For this review, take the finished solid that the model builds, in its own axes (mm). Give positions to 0.01 mm unless a question says otherwise; leave off trailing zeros. Write each loop counter-clockwise with the first axis right and the second up, starting at its lowest first coordinate (ties: lowest second). Pieces come first, ordered by that corner, then holes. Notation, with made-up numbers: M 11.25,38 L 54.25,38 A27 cw 54.25,66 Z; hole C 62,56.5 d9. An arc over 180 degrees is marked long. Write item = value, one per line.
```python
from build123d import *

# Parameters (mm, degrees)
SKETCH_2_W      = 70
SKETCH_2_H      = 70
SKETCH_2_R      = 2.15
EXTRUDE_1_DEPTH = 4
SKETCH_3_R      = 3.5
SKETCH_3_R_2    = 1.5
EXTRUDE_2_DEPTH = 5
FILLET_1_R      = 5


with BuildPart() as part:
    # 草圖2 → 填料-伸長1 (new body)
    with BuildSketch(Plane(origin=(0, 0, 0), x_dir=(1, 0, 0), z_dir=(0, 1, 0))):
        Rectangle(SKETCH_2_W, SKETCH_2_H)
        with Locations(Location((-25, 25, 0), (0, 0, 270))):
            Circle(SKETCH_2_R, mode=Mode.SUBTRACT)
        with Locations(Location((25, 25, 0), (0, 0, 270))):
            Circle(SKETCH_2_R, mode=Mode.SUBTRACT)
        with Locations(Location((-25, -25, 0), (0, 0, 270))):
            Circle(SKETCH_2_R, mode=Mode.SUBTRACT)
        with Locations(Location((25, -25, 0), (0, 0, 270))):
            Circle(SKETCH_2_R, mode=Mode.SUBTRACT)
    extrude(amount=EXTRUDE_1_DEPTH)

    # 草圖3 → 填料-伸長2 (add)
    # profile 1 of 4: a face of its own
    with BuildSketch(Plane(origin=(0, 4, 0), x_dir=(1, 0, 0), z_dir=(0, 1, 0))):
        with Locations(Location((-20, 30, 0), (0, 0, 270))):
            Circle(SKETCH_3_R)
        with Locations(Location((-20, 30, 0), (0, 0, 270))):
            Circle(SKETCH_3_R_2, mode=Mode.SUBTRACT)
    # profile 2 of 4: a face of its own
    with BuildSketch(Plane(origin=(0, 4, 0), x_dir=(1, 0, 0), z_dir=(0, 1, 0))):
        with Locations(Location((30.8, 14.8, 0), (0, 0, 270))):
            Circle(SKETCH_3_R)
        with Locations(Location((30.8, 14.8, 0), (0, 0, 270))):
            Circle(SKETCH_3_R_2, mode=Mode.SUBTRACT)
    # profile 3 of 4: a face of its own
    with BuildSketch(Plane(origin=(0, 4, 0), x_dir=(1, 0, 0), z_dir=(0, 1, 0))):
        with Locations(Location((30.8, -13.1, 0), (0, 0, 270))):
            Circle(SKETCH_3_R)
        with Locations(Location((30.8, -13.1, 0), (0, 0, 270))):
            Circle(SKETCH_3_R_2, mode=Mode.SUBTRACT)
    # profile 4 of 4: a face of its own
    with BuildSketch(Plane(origin=(0, 4, 0), x_dir=(1, 0, 0), z_dir=(0, 1, 0))):
        with Locations(Location((-21.3, -18.2, 0), (0, 0, 270))):
            Circle(SKETCH_3_R)
        with Locations(Location((-21.3, -18.2, 0), (0, 0, 270))):
            Circle(SKETCH_3_R_2, mode=Mode.SUBTRACT)
    extrude(amount=EXTRUDE_2_DEPTH)

    # 圓角1
    fillet_1_edges = [part.edges().sort_by_distance(p)[0] for p in [
        (35, 2, 35),
        (-35, 2, 35),
        (-35, 2, -35),
        (35, 2, -35),
    ]]
    fillet(fillet_1_edges, radius=FILLET_1_R)


solid = part.part
```
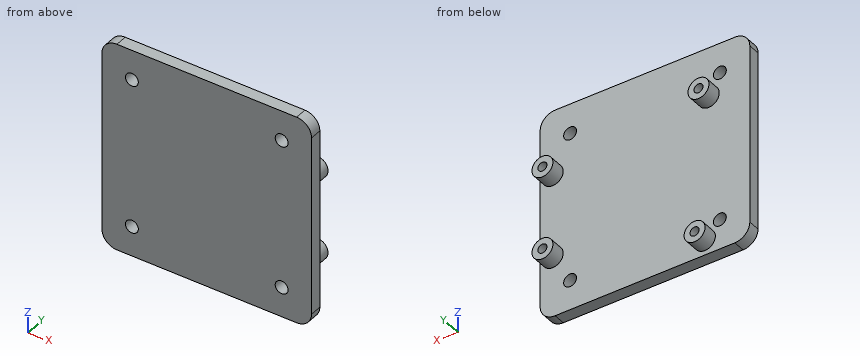
1. We need section C-C, the plane z = -14.8. Write out the cut boundary in (x, y).
Responses:
outline = M -35,0 L 35,0 L 35,4 L 34.3,4 L 34.3,9 L 32.3,9 L 32.3,4 L 29.3,4 L 29.3,9 L 27.3,9 L 27.3,4 L -35,4 Z
2. For line 1 along X through (y, z) = (1.2, -25); line 2 along X through (y, z) = (5.3, -14.8); line 3 along X through (y, z) = (6.9, -30), list the stretches that pass through material, from the lowest coordinate up. Write a range as from..to.
Responses:
line_1 = -35..-27.15, -22.85..22.85, 27.15..35
line_2 = 27.3..29.3, 32.3..34.3
line_3 = -23.5..-21.5, -18.5..-16.5
3. We need section D-D, the plane x = 26. Write out the cut boundary in (y, z).
Responses:
outline = M 0,-35 L 4,-35 L 4,-26.9 L 0,-26.9 Z; M 0,-23.1 L 4,-23.1 L 4,23.1 L 0,23.1 Z; M 0,26.9 L 4,26.9 L 4,35 L 0,35 Z
4. Insertion check: P1, Ø2.5, axis at x = -21.3, z = 18.2, coming from the +Y side; P2, Ø4, axis at y = 6.5, z = -10.5, coming from the -X side; P3, Ø2.5, axis at x = -25, z = 25, coming from the -Y side. Each pin has a flat end and moves straight along its axis. Give the tip position at first contact, or say it passes through.
Responses:
P1 = 4
P2 = 28.16
P3 = through
5. We need section A-A, the plane y = 7.25. Write out the cut boundary in (x, z).
Responses:
outline = C -21.3,18.2 d7; C -20,-30 d7; C 30.8,-14.8 d7; C 30.8,13.1 d7; hole C -21.3,18.2 d3; hole C -20,-30 d3; hole C 30.8,-14.8 d3; hole C 30.8,13.1 d3
6. We need section B-B, the plane z = 25. Write out the cut boundary in (x, y), then the cut area to 3 significant figures.
Responses:
outline = M -35,0 L -27.15,0 L -27.15,4 L -35,4 Z; M -22.85,0 L 22.85,0 L 22.85,4 L -22.85,4 Z; M 27.15,0 L 35,0 L 35,4 L 27.15,4 Z
area = 246 mm2
